The listing builds one solid part. Answer for the finished solid, in the listing's coordinates (mm). Face numbers are marked on the shaded views. A direction names the side the tool comes from. Coordinates: 2 decimals unless noted, no trailing zeros. Loops run counter-clockwise (first coordinate to the right, second up) from the corner with the lowest first, then second, coordinate; pieces in that order, holes last. Notation, with made-up numbers: (55.25, -21.5) -> (112.25, -21.5) arc R21 ccw to (112.25, 14.5) -> close; hole circle Ø10 at (53.25, 1.25). An arc over 180 degrees is marked (long way). Answer in a Markdown table with one row per item.
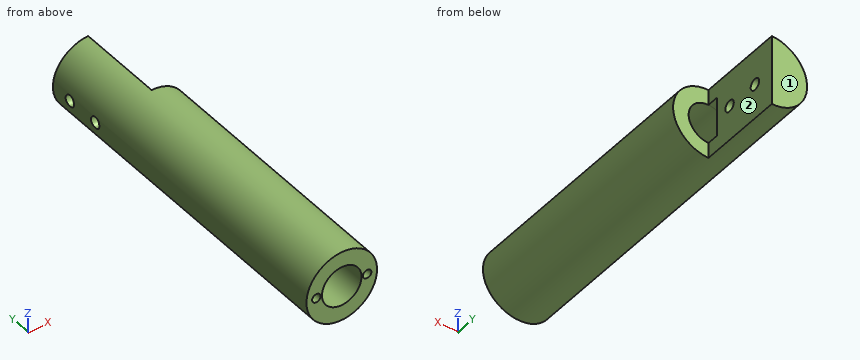
```python
from build123d import *

# Parameters (mm, degrees)
SKETCH1_R           = 6.25
BOSS_EXTRUDE1_DEPTH = 60
CUT_EXTRUDE2_START  = -15
CUT_EXTRUDE2_DEPTH  = 15
SKETCH3_R           = 3.5
CUT_EXTRUDE3_DEPTH  = 46.85984082
CUT_EXTRUDE5_START  = -2
SKETCH7_R           = 3.5
CUT_EXTRUDE5_DEPTH  = 2
SKETCH8_R           = 1
CUT_EXTRUDE6_DEPTH  = 61.647547354
LPATTERN1_COUNT     = 2
LPATTERN1_PITCH     = 6
SKETCH9_R           = 0.75
CUT_EXTRUDE7_DEPTH  = 5
CIRPATTERN1_COUNT   = 2


with BuildPart() as part:
    # Sketch1 → Boss-Extrude1 (new body)
    with BuildSketch(Plane(origin=(0, 0, 0), x_dir=(1, 0, 0), z_dir=(0, 1, 0))):
        with Locations(Location((0, 0, 0), (0, 0, 270))):
            Circle(SKETCH1_R)
    extrude(amount=BOSS_EXTRUDE1_DEPTH)

    # Sketch2 → Cut-Extrude2 (cut)
    with BuildSketch(Plane(origin=(0, 60, 0), x_dir=(1, 0, 0), z_dir=(0, 1, 0)).offset(CUT_EXTRUDE2_START)):
        with BuildLine():
            Line((0, 6.25), (0, -6.25))
            ThreePointArc((0, -6.25), (6.25, 0), (0, 6.25))
        make_face()
    extrude(amount=CUT_EXTRUDE2_DEPTH, mode=Mode.SUBTRACT)

    # Sketch3 → Cut-Extrude3 (cut, through all)
    with BuildSketch(Plane(origin=(0, 45, 0), x_dir=(1, 0, 0), z_dir=(0, 1, 0))):
        with Locations(Location((0, 0, 0), (0, 0, 270))):
            Circle(SKETCH3_R)
    extrude(amount=-CUT_EXTRUDE3_DEPTH, mode=Mode.SUBTRACT)

    # Sketch7 → Cut-Extrude5 (cut)
    with BuildSketch(Plane.XZ.offset(-45).offset(CUT_EXTRUDE5_START)):
        with Locations(Location((0, 0, 0), (0, 0, 90))):
            Circle(SKETCH7_R)
    extrude(amount=CUT_EXTRUDE5_DEPTH, mode=Mode.SUBTRACT)

    # Sketch8 → Cut-Extrude6 (cut, through all)
    with BuildSketch(Plane(origin=(0, 0, 0), x_dir=(0, 0, -1), z_dir=(1, 0, 0))):
        with Locations((0, 56)):
            Circle(SKETCH8_R)
    cut_extrude6 = extrude(amount=-CUT_EXTRUDE6_DEPTH, mode=Mode.SUBTRACT)

    # LPattern1: Cut-Extrude6 ×2
    with Locations(*[(0, -i * LPATTERN1_PITCH, 0) for i in range(1, LPATTERN1_COUNT)]):
        add(cut_extrude6, mode=Mode.SUBTRACT)

    # Sketch9 → Cut-Extrude7 (cut)
    with BuildSketch(Plane.XZ):
        with Locations(Location((-4.5, 0, 0), (0, 0, 270))):
            Circle(SKETCH9_R)
    cut_extrude7 = extrude(amount=-CUT_EXTRUDE7_DEPTH, mode=Mode.SUBTRACT)

    # CirPattern1: Cut-Extrude7 ×2 about axis
    cirpattern1_axis = Axis((0, 0, 0), (0, 1, 0))
    for i in range(1, CIRPATTERN1_COUNT):
        add(cut_extrude7.rotate(cirpattern1_axis, i * 360 / CIRPATTERN1_COUNT), mode=Mode.SUBTRACT)


solid = part.part
```
Item 1: A tool of negligible diameter and unlimited length cuts with its end or side. For the marked faces 1 and 2, from which of +Z, -Z, +X, -X, +Y, -Y can it reach the whole face along a straight path? Write none if from no direction.
Findings below:
| item | result |
|---|---|
| face 1 | +Z, -Z, +X, -X, +Y |
| face 2 | +Z, -Z, +X, +Y |
Item 2: A cutting plane is placed at D-D, the plane x = -4.5. Determine the outline of the cut face in (y, z), plus the area to 3 significant figures.
Findings below:
| item | result |
|---|---|
| outline | (0, -4.34) -> (60, -4.34) -> (60, 4.34) -> (0, 4.34) -> (0, 0.75) -> (5, 0.75) -> (5, -0.75) -> (0, -0.75) -> close; hole circle Ø2 at (50, 0); hole circle Ø2 at (56, 0) |
| area | 507 mm2 |
Item 3: A cutting plane is placed at C-C, the plane y = 35. Determine the outline of the cut face in (x, z).
Findings below:
| item | result |
|---|---|
| outline | circle Ø12.5 at (0, 0); hole circle Ø7 at (0, 0) |
Item 4: A cutting plane is placed at B-B, the plane z = -2.5. Determine the outline of the cut face in (x, y).
Findings below:
| item | result |
|---|---|
| outline | (-5.73, 0) -> (-2.45, 0) -> (-2.45, 47) -> (0, 47) -> (0, 60) -> (-5.73, 60) -> close; (2.45, 0) -> (5.73, 0) -> (5.73, 45) -> (2.45, 45) -> close |
Item 5: A cutting plane is placed at A-A, the plane z = 0. Determine the outline of the cut face in (x, y).
Findings below:
| item | result |
|---|---|
| outline | (-6.25, 0) -> (-5.25, 0) -> (-5.25, 5) -> (-3.75, 5) -> (-3.75, 0) -> (-3.5, 0) -> (-3.5, 47) -> (0, 47) -> (0, 49) -> (-6.25, 49) -> close; (-6.25, 51) -> (0, 51) -> (0, 55) -> (-6.25, 55) -> close; (-6.25, 57) -> (0, 57) -> (0, 60) -> (-6.25, 60) -> close; (3.5, 0) -> (3.75, 0) -> (3.75, 5) -> (5.25, 5) -> (5.25, 0) -> (6.25, 0) -> (6.25, 45) -> (3.5, 45) -> close |
Item 6: Find the intervals of material crossed by probe 1 along Y at (x, z) = (-4.25, 0); probe 2 along X at (y, z) = (2.75, 0); probe 3 along X at (y, z) = (28, 0), in increasing order.
Findings below:
| item | result |
|---|---|
| probe 1 | y = 5 to 49, 51 to 55, 57 to 60 |
| probe 2 | x = -6.25 to -5.25, -3.75 to -3.5, 3.5 to 3.75, 5.25 to 6.25 |
| probe 3 | x = -6.25 to -3.5, 3.5 to 6.25 |
Item 7: Flat-ended cylindrical pins translate along their axes: pin 1 Ø0.9 at (x, z) = (4.5, 0) entering from +Y; pin 2 Ø1.2 at (x, z) = (4.5, 0) entering from -Y; pin 3 Ø3 at (y, z) = (56, 0) entering from +X. Find the tip coordinate at first contact, or state that the pin passes through.
Findings below:
| item | result |
|---|---|
| pin 1 | stops at y = 45 |
| pin 2 | stops at y = 5 |
| pin 3 | stops at x = 0 |
